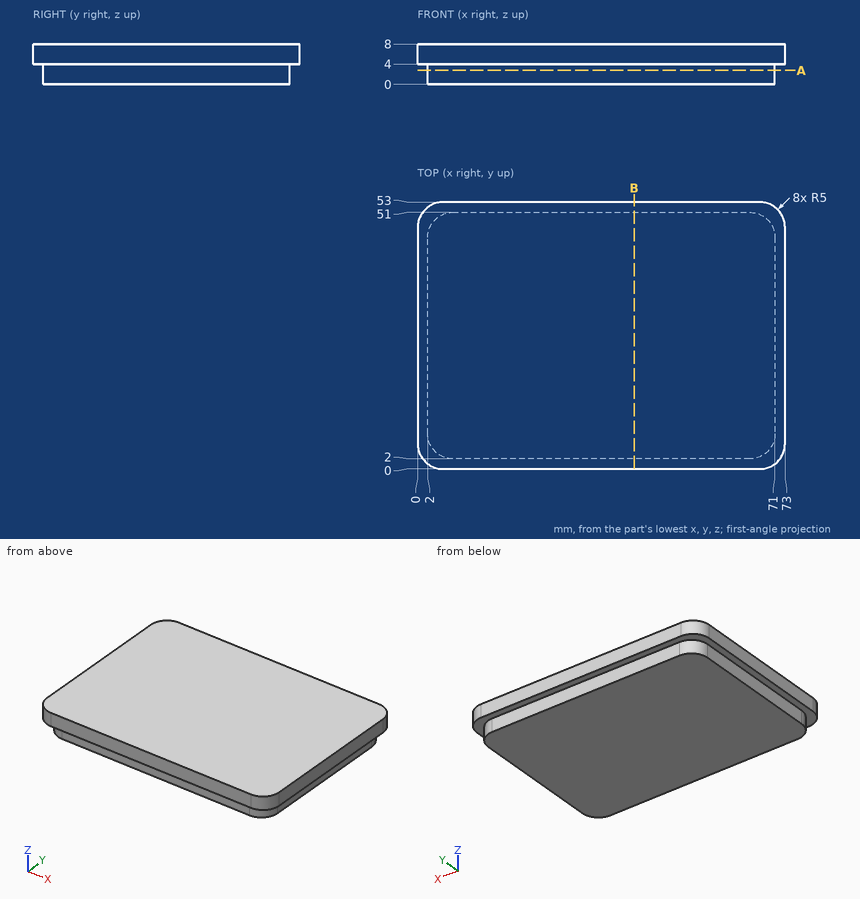
Geometry check sheet. Reference: drawing and pictorial views, mm from the part's lowest x, y, z. Give positions to 0.01 mm unless a question says otherwise; leave off trailing zeros. Order: outer loops, then holes, each group sorted by start corner. A loop starts at its lowest first (then second) coordinate and runs counter-clockwise, first axis right, second up. Notation, with made-up numbers: (19.25, 33) - (24.25, 33) arc R22 ccw to (24.25, 66) - close; hole circle Ø10 at (-8.5, 14). An arc over 180 degrees is marked (long way). Answer as CSV lines item,"result".
1. Scan lines: probe 1 along Y at (x, z) = (43, 1.75); probe 2 along X at (y, z) = (8, 1); probe 3 along Y at (x, z) = (4, 1.5). Record each from-to range of solid material in increasing order. Write a range as from..to.
Result sheet:
probe 1,"2..51"
probe 2,"2..71"
probe 3,"3..50"
2. Section check A-A (z = 2.75). Record the boundary of the cut face in (x, y), then the cut area to 3 significant figures.
Result sheet:
outline,"(2, 7) arc R5 ccw to (7, 2) - (66, 2) arc R5 ccw to (71, 7) - (71, 46) arc R5 ccw to (66, 51) - (7, 51) arc R5 ccw to (2, 46) - close"
area,"3,360 mm²"
3. Go/stop test with flat-tipped pins: P1, Ø1.2, axis at y = 27.5, z = 1, coming from the -X side; P2, Ø2, axis at x = 46.5, z = 1.5, coming from the -Y side; P3, Ø4.5, axis at x = 43.5, z = 1, coming from the +Y side. Record where each tip stops, or that it passes through.
Result sheet:
P1,"x = 2"
P2,"y = 2"
P3,"y = 51"
4. Section check B-B (x = 43). Record the boundary of the cut face in (y, z), then the cut area to 3 significant figures.
Result sheet:
outline,"(0, 4) - (2, 4) - (2, 0) - (51, 0) - (51, 4) - (53, 4) - (53, 8) - (0, 8) - close"
area,"408 mm²"
